Autodesk Inventor part; units mm, degrees
ref_plane "YZ Plane" through (0, 0, 0) normal (1, 0, 0) x (0, 1, 0)
ref_plane "XZ Plane" through (0, 0, 0) normal (0, 1, 0) x (-1, 0, 0)
ref_plane "XY Plane" through (0, 0, 0) normal (0, 0, 1) x (1, 0, 0)
sketch "스케치1" plane through (0, 0, 0) normal (0, 0, 1) x (1, 0, 0)
  line L0 (0, 0) -> (19, 0)
  line L1 (19, 0) -> (19, 75)
  line L2 (19, 75) -> (0, 75)
  line L3 (0, 75) -> (0, 0)
  dimension "d0" = 19
  dimension "d1" = 75
extrude "돌출1" add sketch "스케치1" along normal blind 1.9
sketch "스케치2" plane through (0, 0, 1.9) normal (0, 0, 1) x (1, 0, 0)
  line L0 (2.1, 75) -> (16.9, 75)
  line L1 (16.9, 75) -> (16.9, -1.5)
  line L2 (16.9, -1.5) -> (2.1, -1.5)
  line L3 (2.1, -1.5) -> (2.1, 75)
  line L4 (19, 75) -> (0, 75)
  line L5 (0, 75) -> (0, 0)
  line L6 (19, 0) -> (19, 75)
  dimension "d4" = 0
  dimension "d5" = 2.1
  dimension "d6" = 2.1
  dimension "d7" = 76.5
extrude "돌출2" add sketch "스케치2" along normal blind 2
properties part number "magea"
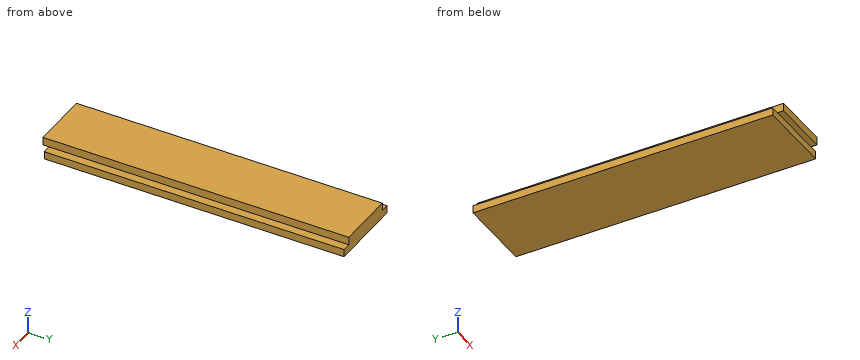
Verification items for the finished model (mm, model axes). Give positions to 0.01 mm unless a question says otherwise; leave off trailing zeros. Order: outer loops, then holes, each group sorted by start corner. A loop starts at its lowest first (then second) coordinate and runs counter-clockwise, first axis right, second up. Notation, with made-up numbers: M 54.25,20 L 81.25,20 A33 cw 81.25,58 Z; hole C 80.25,-16 d6. An arc over 180 degrees is marked long. Answer in a Markdown table with one row per item. Add a question column.
Item 1: Scan lines: probe 1 along X at (y, z) = (50.5, 2.6); probe 2 along Y at (x, z) = (5, 0.4). Record each from-to range of solid material in increasing order. Write a range as from..to.
Item 2: Section check A-A, the plane y = 62. Enter the section's corners in (x, z), and give its area (3 significant figures).
Item 3: Gauge pin test, flat ends, axial feed: pin 1 (1 mm diameter, centred on y = 35, z = 2.5, fed in from -X); pin 2 (0.6 mm diameter, centred on x = 1.5, y = 49.5, fed in from +Z); pin 3 (1 mm diameter, centred on x = 7, z = 1, fed in from -Y). Record the tip position at first contact, or that the pin passes through.
Item 4: Section check B-B, the plane z = 1.3. Enter the section's corners in (x, y), and give its area (4 significant figures).
Filled sheet:
| question | item | result |
|---|---|---|
| 1 | probe 1 | x = 2.1..16.9 |
| 1 | probe 2 | y = 0..75 |
| 2 | outline | M 0,0 L 19,0 L 19,1.9 L 16.9,1.9 L 16.9,3.9 L 2.1,3.9 L 2.1,1.9 L 0,1.9 Z |
| 2 | area | 65.7 mm^2 |
| 3 | pin 1 | stops at x = 2.1 |
| 3 | pin 2 | stops at z = 1.9 |
| 3 | pin 3 | stops at y = 0 |
| 4 | outline | M 0,0 L 19,0 L 19,75 L 0,75 Z |
| 4 | area | 1,425 mm^2 |
